```python
from build123d import *

# Parameters (mm, degrees)
SKETCH_W         = 15.1
SKETCH_H         = 1.7
POCKET_DEPTH     = 5.2
HOLE_D           = 2.7
HOLE_CBORE_D     = 4.7
HOLE_CBORE_DEPTH = 0.7


with BuildPart() as part:
    # Sketch → Revolution (revolve)
    with BuildSketch(Plane.XZ):
        with Locations((16.45, 0.85)):
            Rectangle(SKETCH_W, SKETCH_H)
    revolve(axis=Axis((0, 0, 0), (0, 0, 1)))

    # Sketch001 → Pocket (cut)
    with BuildSketch(Plane.XY.offset(0.3)):
        with BuildLine():
            ThreePointArc((-16.371276, -1.287625), (-19.62355, -4.350436), (-15.381589, -5.751816))
            ThreePointArc((-13.811681, -6.103071), (-14.508018, -5.531376), (-15.381589, -5.751816))
            ThreePointArc((-13.811681, -6.103071), (-13.076984, -7.55), (-12.191255, -8.909731))
            ThreePointArc((-12.672013, -10.444939), (-12.044321, -9.798624), (-12.191255, -8.909731))
            ThreePointArc((-12.672013, -10.444939), (-13.579363, -14.819274), (-9.300754, -13.534129))
            ThreePointArc((-7.813289, -12.921398), (-8.711606, -12.852495), (-9.300754, -13.534129))
            ThreePointArc((-7.813289, -12.921398), (0, -15.1), (7.813289, -12.921398))
            ThreePointArc((9.300754, -13.534129), (8.711606, -12.852495), (7.813289, -12.921398))
            ThreePointArc((9.300754, -13.534129), (13.579363, -14.819274), (12.672013, -10.444939))
            ThreePointArc((12.191255, -8.909731), (12.044321, -9.798624), (12.672013, -10.444939))
            ThreePointArc((12.191255, -8.909731), (13.076984, -7.55), (13.811681, -6.103071))
            ThreePointArc((15.381589, -5.751816), (14.508018, -5.531376), (13.811681, -6.103071))
            ThreePointArc((15.381589, -5.751816), (19.62355, -4.350436), (16.371276, -1.287625))
            ThreePointArc((15.096903, -0.305808), (15.48639, -1.118224), (16.371276, -1.287625))
            ThreePointArc((15.096903, -0.305808), (13.076984, 7.55), (7.283614, 13.227206))
            ThreePointArc((7.070522, 14.821754), (6.774784, 13.970719), (7.283614, 13.227206))
            ThreePointArc((7.070522, 14.821754), (6.044187, 19.169711), (2.709576, 16.196755))
            ThreePointArc((1.620426, 15.012802), (2.463697, 15.33), (2.709576, 16.196755))
            ThreePointArc((1.620426, 15.012802), (0, 15.1), (-1.620426, 15.012802))
            ThreePointArc((-2.709576, 16.196755), (-2.463697, 15.33), (-1.620426, 15.012802))
            ThreePointArc((-2.709576, 16.196755), (-6.044187, 19.169711), (-7.070522, 14.821754))
            ThreePointArc((-7.283614, 13.227206), (-6.774784, 13.970719), (-7.070522, 14.821754))
            ThreePointArc((-7.283614, 13.227206), (-13.076984, 7.55), (-15.096903, -0.305808))
            ThreePointArc((-16.371276, -1.287625), (-15.48639, -1.118224), (-15.096903, -0.305808))
        make_face()
    extrude(amount=POCKET_DEPTH, mode=Mode.SUBTRACT)

    # Hole (through all)
    with Locations(Plane(origin=(0, 0, 0), x_dir=(1, 0, 0), z_dir=(0, 0, -1))):
        with Locations((0, -17.5), (-15.155445, 8.75), (15.155445, 8.75)):
            CounterBoreHole(HOLE_D / 2, HOLE_CBORE_D / 2, HOLE_CBORE_DEPTH)


with BuildPart() as part_1:
    # Clone placement: moved
    add(part.part.moved(Location((0, 0, -1.7))))


solid = part_1.part
```
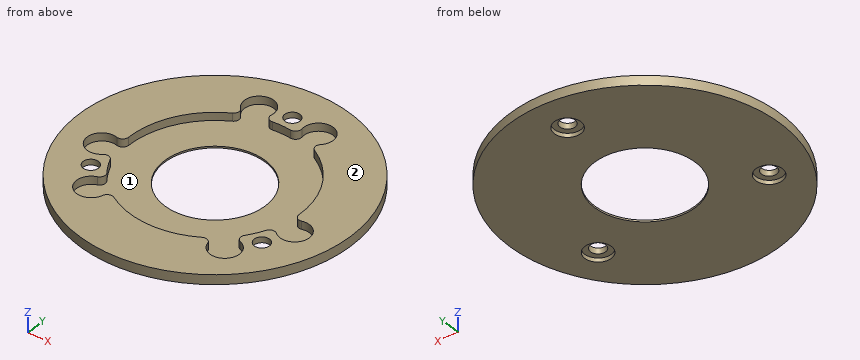
Design review of the part built by this model. Coordinates are the model's own, in mm. Face numbers are marked on the shaded views. Round coordinates to 2 decimals unless told otherwise and drop trailing zeros. Write each loop counter-clockwise with the first axis right and the second up, starting at its lowest first coordinate (ties: lowest second). Pieces come first, ordered by that corner, then holes.
Item 1: For probe 1 along Y at (x, z) = (1, -1.6); probe 2 along X at (y, z) = (-8.75, -0.7); probe 3 along X at (y, z) = (17, -0.9), list the stretches that pass through material, from the lowest coordinate up.
Item 2: We need section D-D on z = -0.3. Write out the cut boundary in (x, y), and give its area (3 significant figures).
Item 3: We need section B-B on y = -8. Write out the cut boundary in (x, z), and give its area (3 significant figures).
Item 4: Clearance check with flat-ended pins moving along their axes: pin 1 Ø3 at (x, y) = (15.16, -8.75) entering from -Z; pin 2 Ø1 at (x, z) = (-15, -1) entering from -Y; pin 3 Ø4 at (x, y) = (17.09, -3.79) entering from +Z. State where each tip first meets the part, or that it passes through.
Item 5: The part is to be moulded in two halves that separate along Y. For the marked faces 1 and 2, say which applies: +Y half, -Y half, draft (parallel to the pull), parting line (faces both ways), or undercut.
Item 6: We need section C-C on y = 17.5. Write out the cut boundary in (x, z), and give its area (3 significant figures).
Item 7: We need section A-A on x = 0. Write out the cut boundary in (y, z).
Returned:
1. probe 1: y = -23.98 to -8.84, 8.84 to 15.37, 19.63 to 23.98
1. probe 2: x = -22.35 to -16.51, -13.81 to -12.31, 12.31 to 13.81, 16.51 to 22.35
1. probe 3: x = -16.94 to -7.84, -2.68 to -1.25, 1.25 to 2.68, 7.84 to 16.94
2. outline: circle Ø48 at (0, 0); hole circle Ø2.7 at (-15.16, -8.75); hole (-16.37, -1.29) arc R2.6 ccw (long way) to (-15.38, -5.75) arc R1 cw to (-13.81, -6.1) arc R15.1 ccw to (-12.19, -8.91) arc R1 cw to (-12.67, -10.44) arc R2.6 ccw (long way) to (-9.3, -13.53) arc R1 cw to (-7.81, -12.92) arc R15.1 ccw to (7.81, -12.92) arc R1 cw to (9.3, -13.53) arc R2.6 ccw (long way) to (12.67, -10.44) arc R1 cw to (12.19, -8.91) arc R15.1 ccw to (13.81, -6.1) arc R1 cw to (15.38, -5.75) arc R2.6 ccw (long way) to (16.37, -1.29) arc R1 cw to (15.1, -0.31) arc R15.1 ccw to (7.28, 13.23) arc R1 cw to (7.07, 14.82) arc R2.6 ccw (long way) to (2.71, 16.2) arc R1 cw to (1.62, 15.01) arc R15.1 ccw to (-1.62, 15.01) arc R1 cw to (-2.71, 16.2) arc R2.6 ccw (long way) to (-7.07, 14.82) arc R1 cw to (-7.28, 13.23) arc R15.1 ccw to (-15.1, -0.31) arc R1 cw to start; hole circle Ø2.7 at (0, 17.5); hole circle Ø2.7 at (15.16, -8.75)
2. area: 942 mm2
3. outline: (-22.63, -1.7) - (-17.38, -1.7) - (-17.38, -1) - (-16.28, -1) - (-16.28, 0) - (-22.63, 0) - close; (-14.03, -1) - (-12.93, -1) - (-12.93, -1.7) - (-3.9, -1.7) - (-3.9, -1.4) - (-12.81, -1.4) - (-12.81, 0) - (-14.03, 0) - close; (3.9, -1.7) - (12.93, -1.7) - (12.93, -1) - (14.03, -1) - (14.03, 0) - (12.81, 0) - (12.81, -1.4) - (3.9, -1.4) - close; (16.28, -1) - (17.38, -1) - (17.38, -1.7) - (22.63, -1.7) - (22.63, 0) - (16.28, 0) - close
3. area: 28.0 mm2
4. pin 1: stops at z = -1
4. pin 2: stops at y = -19.12
4. pin 3: stops at z = -1.4
5. face 1: undercut
5. face 2: draft
6. outline: (-16.42, -1.7) - (-2.35, -1.7) - (-2.35, -1) - (-1.35, -1) - (-1.35, 0) - (-2.79, 0) - (-2.79, -1.4) - (-7.73, -1.4) - (-7.73, 0) - (-16.42, 0) - close; (1.35, -1) - (2.35, -1) - (2.35, -1.7) - (16.42, -1.7) - (16.42, 0) - (7.73, 0) - (7.73, -1.4) - (2.79, -1.4) - (2.79, 0) - (1.35, 0) - close
6. area: 36.0 mm2
7. outline: (-24, -1.7) - (-8.9, -1.7) - (-8.9, -1.4) - (-15.1, -1.4) - (-15.1, 0) - (-24, 0) - close; (8.9, -1.7) - (15.15, -1.7) - (15.15, -1) - (16.15, -1) - (16.15, 0) - (15.1, 0) - (15.1, -1.4) - (8.9, -1.4) - close; (18.85, -1) - (19.85, -1) - (19.85, -1.7) - (24, -1.7) - (24, 0) - (18.85, 0) - close
